Geometry: final body of the model. Coordinates: model frame, mm. Face numbers are marked on the shaded views. Round coordinates to 2 decimals unless told otherwise and drop trailing zeros. Write each loop counter-clockwise with the first axis right and the second up, starting at its lowest first coordinate (ties: lowest second). Pieces come first, ordered by that corner, then holes. Notation, with made-up numbers: (49, -39.5) -> (94, -39.5) arc R13 cw to (94, -30.5) -> close; hole circle Ø10 at (72, -13). An arc over 180 degrees is marked (long way). Use one line per item in the form item = value. Start each with the question number.
1. Draft query along X for the marked faces 1 and 2. Return one class per face: pulls with the +X half, pulls with the -X half, needs draft (parallel to the pull), parting line crosses it, or undercut.
2. Cut plane D-D, the plane x = 79. Return the cut outline in (y, z), plus the area to 3 significant figures.
3. Line query: L1, parallel to Y at x = 36.5, z = 73.5; L2, parallel to Z at x = 74, y = 4.25; L3, parallel to Z at x = 22.5, y = 6.25. Output: solid intervals per line, ascending.
4. Pin query (flat end, axial travel): pin 1 Ø3 at (x, z) = (14.5, 32) entering from -Y; pin 2 Ø3.5 at (x, z) = (73.09, 12) entering from +Y; pin 3 Ø12 at (x, z) = (72.5, 42) entering from +Y; pin 4 Ø5 at (x, z) = (2.09, 83) entering from +Y. Return the tip coordinate at first contact, or that it passes through.
5. Cut plane C-C, the plane z = 12. Return the cut outline in (x, y), plus the area to 3 significant figures.
6. Cut plane B-B, the plane x = 14. Return the cut outline in (y, z), plus the area to 3 significant figures.
7. Cut plane A-A, the plane z = 47.5. Return the cut outline in (x, y), plus the area to 3 significant figures.
Autodesk Inventor part; units mm, degrees
ref_plane "Work Plane1" through (0, 15, 0) normal (0, 1, 0) x (-1, 0, 0)
ref_plane "YZ Plane" through (0, 0, 0) normal (1, 0, 0) x (0, 1, 0)
ref_plane "XY Plane" through (0, 0, 0) normal (0, 0, 1) x (1, 0, 0)
sketch "Sketch1" plane through (0, 0, 0) normal (0, 0, 1) x (1, 0, 0)
  arc A0 (85.0917, -2.3076) -> (-9.9083, -2.3076) centre (37.5917, -117.9309) ccw
  arc A1 (85.0917, 2.8037) -> (-9.9083, 2.8037) centre (37.5917, -101.9281) ccw
  line L0 (-9.9083, -2.3076) -> (-9.9083, 2.8037)
  line L1 (85.0917, -2.3076) -> (85.0917, 2.8037)
  point P0 (0, 0)
extrude "Extrusion1" add sketch "Sketch1" along normal blind 95
sketch "Sketch2" plane through (0, 0, 0) normal (0, 1, 0) x (-1, 0, 0)
  line L0 (12.4083, 0) -> (12.4083, 95)
  line L1 (-85.0917, 95) -> (9.9083, 95)
  line L2 (9.9083, 0) -> (-85.0917, 0)
  line L3 (-87.5917, 0) -> (-87.5917, 95)
  line L4 (9.9083, 0) -> (9.9083, 95)
  line L5 (-85.0917, 0) -> (-85.0917, 95)
  point P0 (0, 0)
  point P1 (-2.0917, 83)
  point P2 (-2.0917, 12)
  point P3 (-73.0917, 12)
  point P4 (-73.0917, 83)
  dimension "d14" = 12
  dimension "d30" = 12
  dimension "d31" = 12
  dimension "d32" = 12
  dimension "d33" = 12
  dimension "d34" = 12
  dimension "d35" = 12
  dimension "d37" = 12
ref_plane "Work Plane1" through (0, 15, 0) normal (0, 1, 0) x (-1, 0, 0)
sketch "Sketch3" plane through (0, 15, 0) normal (0, 1, 0) x (-1, 0, 0)
  point P0 (0, 0)
  point P1 (-2.0917, 12)
  point P2 (-2.0917, 83)
  point P3 (-73.0917, 83)
  point P4 (-73.0917, 12)
hole "Hole1" at (73.0917, 15, 83) at (2.0917, 15, 83) at (2.0917, 15, 12) at (73.0917, 15, 12) direction (0, -1, 0) diameter 4.5 depth 34.9875 tip angle 118
sketch "Sketch4" plane through (0, 15, 0) normal (0, 1, 0) x (-1, 0, 0)
  line L0 (9.9083, 0) -> (-85.0917, 0)
  circle A0 centre (-37.5917, 47.5) radius 25.4
  line L1 (-85.0917, 0) -> (-85.0917, 95)
  point P0 (0, 0)
  dimension "d23" = 47.5
  dimension "d25" = 50.8
  dimension "d36" = 47.5
extrude "Extrusion2" cut sketch "Sketch4" against normal blind 24.2875
properties part number "dopasowywacz" material "ABS Plastic"
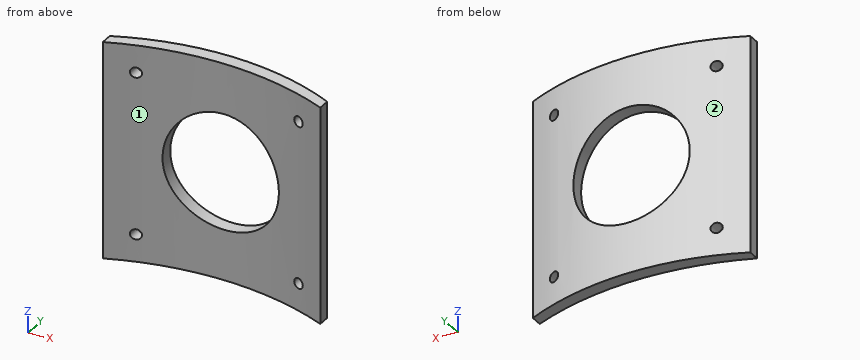
Outcome:
q1.face_1 = undercut
q1.face_2 = parting line crosses it
q2.outline = (0.01, 0) -> (5.36, 0) -> (5.36, 95) -> (0.01, 95) -> close
q2.area = 508 mm^2
q3.L1 = 7.06 to 13.07
q3.L2 = 0 to 9.94, 14.06 to 80.94, 85.06 to 95
q3.L3 = 0 to 27.07, 67.93 to 95
q4.pin_1 = 4.63
q4.pin_2 = through
q4.pin_3 = 9.38
q4.pin_4 = 8.23
q5.outline = (-9.91, -2.31) arc R125 cw to (-0.16, 1.23) -> (-0.16, 6.7) arc R115 ccw to (-9.91, 2.8) -> close; (4.34, 2.57) arc R125 cw to (70.84, 2.57) -> (70.84, 8.16) arc R115 ccw to (4.34, 8.16) -> close; (75.34, 1.23) arc R125 cw to (85.09, -2.31) -> (85.09, 2.8) arc R115 ccw to (75.34, 6.7) -> close
q5.area = 494 mm^2
q6.outline = (4.82, 0) -> (10.63, 0) -> (10.63, 38.09) -> (4.82, 38.09) -> close; (4.82, 56.91) -> (10.63, 56.91) -> (10.63, 95) -> (4.82, 95) -> close
q6.area = 442 mm^2
q7.outline = (-9.91, -2.31) arc R125 cw to (12.19, 4.46) -> (12.19, 10.23) arc R115 ccw to (-9.91, 2.8) -> close; (62.99, 4.46) arc R125 cw to (85.09, -2.31) -> (85.09, 2.8) arc R115 ccw to (62.99, 10.23) -> close
q7.area = 242 mm^2
